Geometry check sheet. Reference: the model listing, model coordinates, mm. A direction names the side the tool comes from. Give positions to 0.01 mm unless a question says otherwise; leave off trailing zeros. Order: outer loops, then holes, each group sorted by start corner. A loop starts at its lowest first (then second) coordinate and runs counter-clockwise, first axis right, second up.
from build123d import *

# Parameters (mm, degrees)
SKETCH1_W           = 20
SKETCH1_H           = 20
BOSS_EXTRUDE1_DEPTH = 7
SKETCH4_W           = 4
SKETCH4_H           = 20
BOSS_EXTRUDE2_DEPTH = 10
BOSS_EXTRUDE3_DEPTH = 4
BOSS_EXTRUDE4_START = -4
BOSS_EXTRUDE4_DEPTH = 4
SKETCH7_R           = 0.85
CUT_EXTRUDE1_DEPTH  = 31
FILLET1_R           = 4
SKETCH8_W           = 4
SKETCH8_H           = 20
BOSS_EXTRUDE5_DEPTH = 10
SKETCH9_R           = 10
BOSS_EXTRUDE6_DEPTH = 4
BOSS_EXTRUDE7_START = -4
SKETCH10_R          = 10
BOSS_EXTRUDE7_DEPTH = 4
SKETCH12_R          = 1.1
CUT_EXTRUDE2_DEPTH  = 33.939338184
SKETCH13_R          = 6
BOSS_EXTRUDE8_DEPTH = 4
SKETCH14_R          = 1.1
CUT_EXTRUDE3_DEPTH  = 4
FILLET2_R           = 2
CUT_EXTRUDE4_REACH  = 32.48
SKETCH16_R          = 0.5


with BuildPart() as part:
    # Sketch1 → Boss-Extrude1 (new body)
    with BuildSketch(Plane(origin=(0, 0, 0), x_dir=(1, 0, 0), z_dir=(0, 1, 0))):
        Rectangle(SKETCH1_W, SKETCH1_H)
    extrude(amount=BOSS_EXTRUDE1_DEPTH)

    # Sketch4 → Boss-Extrude2 (add)
    with BuildSketch(Plane.XZ):
        with Locations((-8, 0)):
            Rectangle(SKETCH4_W, SKETCH4_H)
        with Locations((8, 0)):
            Rectangle(SKETCH4_W, SKETCH4_H)
    extrude(amount=BOSS_EXTRUDE2_DEPTH)

    # Sketch5 → Boss-Extrude3 (add)
    with BuildSketch(Plane.ZY.offset(10)):
        with BuildLine():
            Line((0, -20), (10, -20))
            Line((10, -20), (10, -10))
            ThreePointArc((10, -10), (-7.071067812, -2.928932188), (0, -20))
        make_face()
    extrude(amount=-BOSS_EXTRUDE3_DEPTH)

    # Sketch6 → Boss-Extrude4 (add)
    with BuildSketch(Plane(origin=(10, 0, 0), x_dir=(0, 0, -1), z_dir=(1, 0, 0)).offset(BOSS_EXTRUDE4_START)):
        with BuildLine():
            Line((0, -20), (-10, -20))
            Line((-10, -20), (-10, -10))
            ThreePointArc((-10, -10), (7.071067812, -2.928932188), (0, -20))
        make_face()
    extrude(amount=BOSS_EXTRUDE4_DEPTH)

    # Sketch7 → Cut-Extrude1 (cut, through all)
    with BuildSketch(Plane.ZY.offset(10)):
        with Locations((0, -10)):
            Circle(SKETCH7_R)
    extrude(amount=-CUT_EXTRUDE1_DEPTH, mode=Mode.SUBTRACT)

    # Fillet1
    fillet1_edges = [part.edges().sort_by_distance(p)[0] for p in [
        (-10, -6.5, 10),
        (-10, -17.071067812, -7.071067812),
        (10, -6.5, 10),
        (10, -17.071067812, -7.071067812),
        (-10, -1.5, -10),
        (10, -1.5, -10),
        (10, -20, 5),
        (-10, -20, 5),
    ]]
    fillet(fillet1_edges, radius=FILLET1_R - 0.0001)  # a hair under: the kernel refuses the full size

    # Sketch8 → Boss-Extrude5 (add)
    with BuildSketch(Plane(origin=(0, 7, 0), x_dir=(1, 0, 0), z_dir=(0, 1, 0))):
        with Locations((4, 0)):
            Rectangle(SKETCH8_W, SKETCH8_H)
        with Locations((-4, 0)):
            Rectangle(SKETCH8_W, SKETCH8_H)
    extrude(amount=BOSS_EXTRUDE5_DEPTH)

    # Sketch9 → Boss-Extrude6 (add)
    with BuildSketch(Plane(origin=(6, 0, 0), x_dir=(0, 0, -1), z_dir=(1, 0, 0))):
        with Locations((0, 17)):
            Circle(SKETCH9_R)
    extrude(amount=-BOSS_EXTRUDE6_DEPTH)

    # Sketch10 → Boss-Extrude7 (add)
    with BuildSketch(Plane.ZY.offset(6).offset(BOSS_EXTRUDE7_START)):
        with Locations((0, 17)):
            Circle(SKETCH10_R)
    extrude(amount=BOSS_EXTRUDE7_DEPTH)

    # Sketch12 → Cut-Extrude2 (cut, through all)
    with BuildSketch(Plane.ZY.offset(6)):
        with Locations((0, 17)):
            Circle(SKETCH12_R)
    extrude(amount=-CUT_EXTRUDE2_DEPTH, mode=Mode.SUBTRACT)

    # Sketch13 → Boss-Extrude8 (add)
    with BuildSketch(Plane(origin=(-2, 0, 0), x_dir=(0, 0, -1), z_dir=(1, 0, 0))):
        with Locations(Location((0, 17, 0), (0, 0, 180))):
            Circle(SKETCH13_R)
    extrude(amount=BOSS_EXTRUDE8_DEPTH)

    # Sketch14 → Cut-Extrude3 (cut)
    with BuildSketch(Plane(origin=(-2, 0, 0), x_dir=(0, 0, -1), z_dir=(1, 0, 0))):
        with Locations(Location((0, 17, 0), (0, 0, 180))):
            Circle(SKETCH14_R)
    extrude(amount=CUT_EXTRUDE3_DEPTH, mode=Mode.SUBTRACT)

    # Fillet2
    fillet2_edges = [part.edges().sort_by_distance(p)[0] for p in [
        (-2, 17, -6),
        (2, 17, -6),
    ]]
    fillet(fillet2_edges, radius=FILLET2_R - 0.0001)  # a hair under: the kernel refuses the full size

    # Sketch16 → Cut-Extrude4 (cut, up to next)
    with BuildSketch(Plane.XZ, mode=Mode.PRIVATE) as cut_extrude4_sk1:
        with Locations(Location((0, -6, 0), (0, 0, 270))):
            Circle(SKETCH16_R)
    cut_extrude4_tool1 = extrude(cut_extrude4_sk1.sketch, amount=-CUT_EXTRUDE4_REACH, mode=Mode.PRIVATE) & part.part
    # Sketch16 → Cut-Extrude4 (cut, up to next)
    with BuildSketch(Plane.XZ, mode=Mode.PRIVATE) as cut_extrude4_sk2:
        with Locations(Location((0, 6, 0), (0, 0, 90))):
            Circle(SKETCH16_R)
    cut_extrude4_tool2 = extrude(cut_extrude4_sk2.sketch, amount=-CUT_EXTRUDE4_REACH, mode=Mode.PRIVATE) & part.part
    add(cut_extrude4_tool1.solids().sort_by_distance((0, 0, -6))[0], mode=Mode.SUBTRACT)
    add(cut_extrude4_tool2.solids().sort_by_distance((0, 0, 6))[0], mode=Mode.SUBTRACT)


solid = part.part
Item 1: Sectioned sample at B-B (x = 4). Enter the section's corners in (y, z).
Reported:
outline: (0, -10) - (17, -10) arc R10 ccw to (17, 10) - (0, 10) - close; hole circle Ø2.2 at (17, 0)
Item 2: Scan lines: L1, parallel to Y at x = -2.5, z = 0; L2, parallel to X at y = -1, z = -5; L3, parallel to Y at x = 0.75, z = 0. Record each from-to range of solid material in increasing order.
Reported:
L1: y = 0 to 15.9, 18.1 to 27
L2: x = -10 to -6, 6 to 10
L3: y = 0 to 7, 10.85 to 15.9, 18.1 to 23.15
Item 3: Gauge pin test, flat ends, axial feed: pin 1 (1.5 mm diameter, centred on x = -2, z = -5.5, fed in from -Y); pin 2 (1.2 mm diameter, centred on x = -9, z = 0.5, fed in from +Y); pin 3 (8 mm diameter, centred on y = 19, z = 5, fed in from -X). Record the tip position at first contact, or that the pin passes through.
Reported:
pin 1: stops at y = 0
pin 2: stops at y = 7
pin 3: stops at x = -6
Item 4: Set-up check for faces 4 (the flat face through (-2, 10, 5)), 5 (the cylindrical face through (-8.859, -18.797, 3.959)), 6 (the flat face through (6, -10, 2)), 7 (the flat face through (8, 7, 0)), 8 (the cylindrical face through (0.3, 3.5, 5.6)): record each of +Z, -Z, +X, -X, +Y, -Y from which the full face is reachable in a straight line by a thin tool's end or side.
Reported:
face 4: none
face 5: +Z, -Z, -X, -Y
face 6: +Z, -Z, -Y
face 7: +Z, -Z, +X, +Y
face 8: -Y
Item 5: Sectioned sample at A-A (y = 5). Enter the section's corners in (x, z), and give its area (3 significant figures).
Reported:
outline: (-10, -6) arc R4 ccw to (-6, -10) - (6, -10) arc R4 ccw to (10, -6) - (10, 6) arc R4 ccw to (6, 10) - (-6, 10) arc R4 ccw to (-10, 6) - close; hole circle Ø1 at (0, -6); hole circle Ø1 at (0, 6)
area: 385 mm2
Item 6: Sectioned sample at C-C (x = 7.25). Enter the section's corners in (y, z).
Reported:
outline: (-19.8, 0) arc R9.8 ccw to (-10, -9.8) - (7, -9.8) - (7, 9.8) - (-19.8, 9.8) - close; hole circle Ø1.7 at (-10, 0)
Item 7: Draft check along Z on faces 1 (the flat face through (-0.1, 6.7, -10)), 2 (the flat face through (10, -4, 0)), 3 (the cylindrical face through (-0.3, 3.5, -5.6)). Enter one of: released by +Z, released by -Z, zero draft, split by the parting line, or undercut.
Reported:
face 1: released by -Z
face 2: zero draft
face 3: undercut
